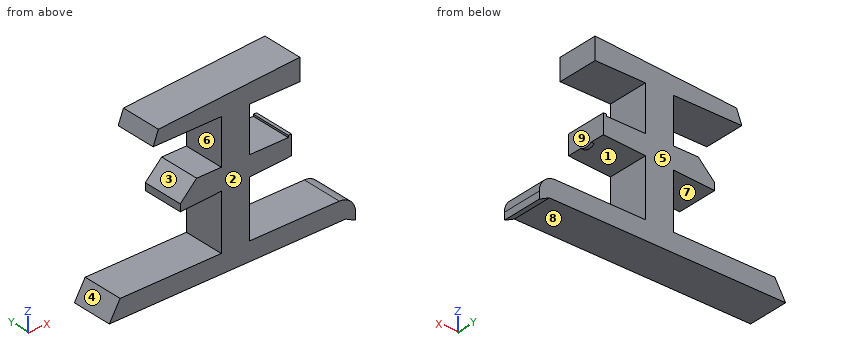
```python
from build123d import *

# Parameters (mm, degrees)
F0_W     = 8.7596660014
F0_H     = 13.9908213168
F0_W_2   = 0.9912690148
F0_H_2   = 0.5951654166
F1_DEPTH = 6.35
F2_R     = 5.08
F4_SIZE  = 5.08


with BuildPart() as f1:
    # F0 (on Front) → F1 (new body, symmetric)
    with BuildSketch(Plane.XZ):
        Polygon((18.4732656926, 41.3089023039), (-25.4520159215, 38.7587957084), (-27.0884726197, 34.5398373902), (-25.4520159215, 34.5398373902), (-5.9040691704, 34.5398373902), (2.8555968311, 34.5398373902), (18.4732656926, 34.5398373902), align=None)
        with Locations((-1.5242361696, 27.5444267318)):
            Rectangle(F0_W, F0_H)
        Polygon((14.8897180334, 20.5490160733), (2.8555968311, 20.5490160733), (2.8555968311, 17.8197465704), (15.8809870481, 17.8197465704), (15.8809870481, 20.5490160733), align=None)
        Polygon((2.8555968311, 17.8197465704), (2.8555968311, 20.5490160733), (-5.9040691704, 20.5490160733), (-5.9040691704, 13.9371497284), (2.8555968311, 14.4008970871), align=None)
        Polygon((-5.9040691704, 13.9371497284), (-5.9040691704, 20.5490160733), (-18.6544265598, 20.5490160733), (-18.6544265598, 13.2621303201), align=None)
        Polygon((15.8809870481, 17.8197465704), (2.8555968311, 17.8197465704), (2.8555968311, 14.4008970871), (15.8809870481, 15.0904770675), align=None)
        with Locations((15.3853525408, 20.8465987816)):
            Rectangle(F0_W_2, F0_H_2)
        Polygon((2.8555968311, 14.4008970871), (-5.9040691704, 13.9371497284), (-5.9040691704, -3.2693331596), (-37.3304970562, -3.2693331596), (-40.6903134995, -9.0090157464), (32.6927527785, -9.0090157464), (35.8047001064, -10.5649875477), (35.8047001064, -3.2693331596), (2.8555968311, -3.2693331596), align=None)
    extrude(amount=F1_DEPTH, both=True)

    # F2
    f2_edges = [f1.edges().sort_by_distance(p)[0] for p in [
        (35.8047, 0, -3.269333),
    ]]
    fillet(f2_edges, radius=F2_R)

    # F0 (on Front) → F3 (revolve)
    with BuildSketch(Plane.XZ):
        with Locations((15.3853525408, 20.8465987816)):
            Rectangle(F0_W_2, F0_H_2)
    revolve(axis=Axis((9.3682919396, 0, 17.8197465704), (-1, 0, 0)))

    # F4
    f4_edges = [f1.edges().sort_by_distance(p)[0] for p in [
        (-18.654427, 0, 20.549016),
    ]]
    chamfer(f4_edges, length=F4_SIZE)


solid = f1.part
```
Geometry: final body of the model. Coordinates: model frame, mm. Face numbers are marked on the shaded views. A direction names the side the tool comes from. Give positions to 0.01 mm unless a question says otherwise; leave off trailing zeros. Write each loop counter-clockwise with the first axis right and the second up, starting at its lowest first coordinate (ties: lowest second). Pieces come first, ordered by that corner, then holes.
1. Draft query along Z for the marked faces 1, 2, 3 and 4. Return one class per face: released by +Z, released by -Z, zero draft, split by the parting line, or undercut.
2. Section query D-D, the plane z = 30. Return loops of the section in (x, y), then the cut area to 3 significant figures.
3. Section query B-B, the plane y = 0. Return loops of the section in (x, z), then the cut area to 3 significant figures.
4. Section query C-C, the plane x = -23. Return loops of the section in (y, z), then the cut area to 3 significant figures.
5. Reachability of the marked faces 5, 6, 7, 8 and 9 from +Z, -Z, +X, -X, +Y, -Y: full face, straight path, thin tool, end or side. Return the list, or none.
6. Line query: probe 1 along Z at (x, y) = (5, 4); probe 2 along Z at (x, y) = (-13.5, 2.5); probe 3 along X at (y, z) = (-2.25, -2). Output: solid intervals per line, ascending.
7. Section query A-A, the plane x = -11. Return loops of the section in (y, z), then the cut area to 3 significant figures.
8. Pin query (flat end, axial travel): P1, Ø6.5, axis at x = -18.5, y = -1, coming from the +Z side; P2, Ø5.5, axis at y = -1.5, z = 38, coming from the +X side; P3, Ø6, axis at x = 10, z = 30, coming from the -Y side; P4, Ø5, axis at y = -2.5, z = 26, coming from the +X side. Return the tip coordinate at first contact, or that it passes through.
Computed:
1. face 1: undercut
1. face 2: zero draft
1. face 3: undercut
1. face 4: released by +Z
2. outline: (-5.9, -6.35) - (2.86, -6.35) - (2.86, 6.35) - (-5.9, 6.35) - close
2. area: 111 mm2
3. outline: (-40.69, -9.01) - (32.69, -9.01) - (35.8, -10.56) - (35.8, -8.35) arc R5.08 ccw to (30.72, -3.27) - (2.86, -3.27) - (2.86, 14.4) - (14.89, 15.04) - (14.89, 14.5) - (15.88, 14.5) - (15.88, 21.14) - (14.89, 21.14) - (14.89, 20.55) - (2.86, 20.55) - (2.86, 34.54) - (18.47, 34.54) - (18.47, 41.31) - (-25.45, 38.76) - (-27.09, 34.54) - (-5.9, 34.54) - (-5.9, 20.55) - (-13.57, 20.55) - (-18.65, 15.47) - (-18.65, 13.26) - (-5.9, 13.94) - (-5.9, -3.27) - (-37.33, -3.27) - close
3. area: 1,150 mm2
4. outline: (-6.35, -9.01) - (6.35, -9.01) - (6.35, -3.27) - (-6.35, -3.27) - close; (-6.35, 34.54) - (6.35, 34.54) - (6.35, 38.9) - (-6.35, 38.9) - close
4. area: 128 mm2
5. face 5: +Z, -Z, +X, -X, +Y
5. face 6: -X, +Y, -Y
5. face 7: +Y, -Y
5. face 8: -Z, -X, +Y, -Y
5. face 9: +X, +Y, -Y
6. probe 1: z = -9.01 to -3.27, 14.51 to 20.55, 34.54 to 40.53
6. probe 2: z = -9.01 to -3.27, 13.54 to 20.55, 34.54 to 39.45
6. probe 3: x = -5.9 to 2.86
7. outline: (-6.35, -9.01) - (6.35, -9.01) - (6.35, -3.27) - (-6.35, -3.27) - close; (-6.35, 13.67) - (6.35, 13.67) - (6.35, 20.55) - (-6.35, 20.55) - close; (-6.35, 34.54) - (6.35, 34.54) - (6.35, 39.6) - (-6.35, 39.6) - close
7. area: 225 mm2
8. P1: stops at z = 39.35
8. P2: stops at x = 18.47
8. P3: passes through
8. P4: stops at x = 2.86
